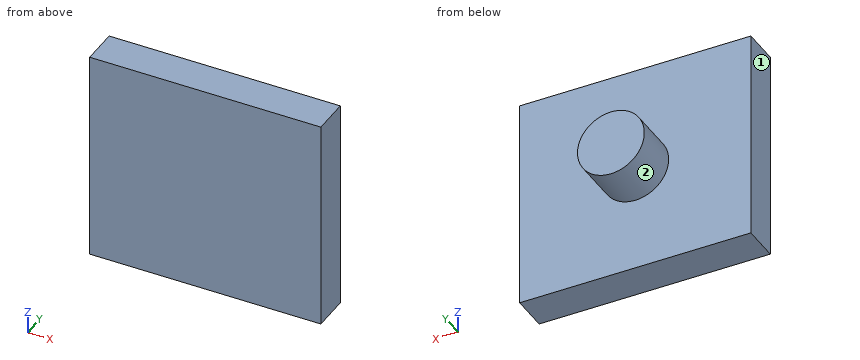
Autodesk Inventor part; units mm, degrees
ref_plane "YZ Plane" through (0, 0, 0) normal (1, 0, 0) x (0, 1, 0)
ref_plane "XZ Plane" through (0, 0, 0) normal (0, 1, 0) x (-1, 0, 0)
ref_plane "XY Plane" through (0, 0, 0) normal (0, 0, 1) x (1, 0, 0)
sketch "Sketch1" plane through (0, 0, 0) normal (0, 1, 0) x (-1, 0, 0)
  line L0 (25, 23) -> (0, 23)
  line L1 (0, 23) -> (0, 0)
  line L2 (0, 0) -> (25, 0)
  line L3 (25, 0) -> (25, 23)
  dimension "d0" = 25
  dimension "d1" = 23
extrude "Extrusion1" add sketch "Sketch1" along normal blind 4
sketch "Sketch2" plane through (0, 4, 0) normal (0, 1, 0) x (1, 0, 0)
  circle A0 centre (-12.5, -11.5) radius 3.615
  line L0 (-25, 0) -> (-25, -23)
  line L1 (-25, -23) -> (0, -23)
  point P0 (0, 0)
  dimension "d4" = 7.23
  dimension "d5" = 12.5
  dimension "d6" = 11.5
extrude "Extrusion2" add sketch "Sketch2" along normal blind 5
properties part number "Camera" material "ABS Plastic"
Work out the finished part from the listing and answer in its coordinate system (mm). Face numbers are marked on the shaded views. A direction names the side the tool comes from. Round coordinates to 2 decimals unless told otherwise and drop trailing zeros. Write each loop counter-clockwise with the first axis right and the second up, starting at its lowest first coordinate (ties: lowest second). Pieces come first, ordered by that corner, then holes.
1) A cutting plane is placed at D-D on z = 20. Determine the outline of the cut face in (x, y).
2) A cutting plane is placed at B-B on z = 11.5. Determine the outline of the cut face in (x, y) (3 decimals).
3) Consider probe 1 along Y at (x, z) = (-21.25, 3.75); probe 2 along Z at (x, y) = (-14.5, 7); probe 3 along Z at (x, y) = (-11, 8). Determine where each line is inside the solid, lowest interval first.
4) A cutting plane is placed at C-C on y = 4.5. Determine the outline of the cut face in (x, z) (3 decimals).
5) Which of the six approach directions +Z, -Z, +X, -X, +Y, -Y give full straight-line access (tool end or side, diameter ignored) to the marked faces 1 and 2?
6) A cutting plane is placed at A-A on x = -12.5. Determine the outline of the cut face in (y, z) (3 decimals), and give its area (3 significant figures).
Entries:
1. outline: (-25, 0) - (0, 0) - (0, 4) - (-25, 4) - close
2. outline: (-25, 0) - (0, 0) - (0, 4) - (-8.885, 4) - (-8.885, 9) - (-16.115, 9) - (-16.115, 4) - (-25, 4) - close
3. probe 1: y = 0 to 4
3. probe 2: z = 8.49 to 14.51
3. probe 3: z = 8.21 to 14.79
4. outline: circle Ø7.23 at (-12.5, 11.5)
5. face 1: +Z, -Z, -X, +Y, -Y
5. face 2: +Y
6. outline: (0, 0) - (4, 0) - (4, 7.885) - (9, 7.885) - (9, 15.115) - (4, 15.115) - (4, 23) - (0, 23) - close
6. area: 128 mm2
